```python
from build123d import *

# Parameters (mm, degrees)
SKETCH2_W           = 100
SKETCH2_H           = 72
BOSS_EXTRUDE1_DEPTH = 6.35
FILLET1_R           = 8
SKETCH4_R           = 6.25
SKETCH4_R_2         = 4
SKETCH4_R_3         = 3.15
SKETCH4_R_4         = 1.25
CUT_EXTRUDE9_DEPTH  = 124.386881393
SKETCH5_R           = 1.65
CUT_EXTRUDE11_DEPTH = 124.386881393
CHAMFER1_SIZE       = 1.5


with BuildPart() as part:
    # Sketch2 → Boss-Extrude1 (new body)
    with BuildSketch(Plane.XY):
        with Locations((50, 36)):
            Rectangle(SKETCH2_W, SKETCH2_H)
    extrude(amount=BOSS_EXTRUDE1_DEPTH)

    # Fillet1
    fillet1_edges = [part.edges().sort_by_distance(p)[0] for p in [
        (100, 0, 3.175),
        (0, 0, 3.175),
    ]]
    fillet(fillet1_edges, radius=FILLET1_R)

    # Sketch4 → Cut-Extrude9 (cut, through all)
    with BuildSketch(Plane.XY):
        with Locations((17.5, 14)):
            Circle(SKETCH4_R)
        with Locations((82.5, 14)):
            Circle(SKETCH4_R_2)
        with Locations((20, 57)):
            Circle(SKETCH4_R_3)
        with Locations((80, 57)):
            Circle(SKETCH4_R_3)
        with Locations((10, 45)):
            Circle(SKETCH4_R_4)
        with Locations((25, 45)):
            Circle(SKETCH4_R_4)
    extrude(amount=CUT_EXTRUDE9_DEPTH, mode=Mode.SUBTRACT)

    # Sketch5 → Cut-Extrude11 (cut, through all)
    with BuildSketch(Plane.XY.offset(6.35)):
        with Locations((10.126311132, 29.325110598)):
            Circle(SKETCH5_R)
        with Locations((36.565235622, 24.663214869)):
            Circle(SKETCH5_R)
        with Locations((19.308453246, 4.097382476)):
            Circle(SKETCH5_R)
    extrude(amount=-CUT_EXTRUDE11_DEPTH, mode=Mode.SUBTRACT)

    # Chamfer1
    chamfer1_edges = [part.edges().sort_by_distance(p)[0] for p in [
        (8.476311132, 29.325110598, 0),
        (8.476311132, 29.325110598, 6.35),
        (34.915235622, 24.663214869, 0),
        (34.915235622, 24.663214869, 6.35),
        (17.658453246, 4.097382476, 0),
        (17.658453246, 4.097382476, 6.35),
    ]]
    chamfer(chamfer1_edges, length=CHAMFER1_SIZE)


solid = part.part
```
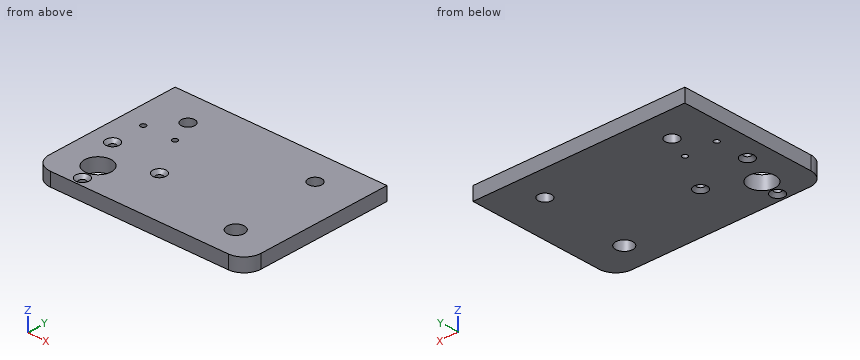
Geometry check sheet. Reference: the model listing, model coordinates, mm. Coordinates: 2 decimals unless noted, no trailing zeros. Order: outer loops, then holes, each group sorted by start corner. A loop starts at its lowest first (then second) coordinate and runs counter-clockwise, first axis right, second up. Notation, with made-up numbers: M 56.25,62 L 113.25,62 A20 ccw 113.25,98 Z; hole C 50.5,53 d3. An arc over 180 degrees is marked long. One line per question, with ' | ' between items. Start each with the question number.
Item 1: Material ranges on L1, parallel to X at y = 14, z = 4; L2, parallel to X at y = 57, z = 4.5; L3, parallel to Y at x = 10, z = 3.25, recorded low to high. Write a range as [from, to].
Item 2: Cross-section at C-C on z = 2.75. State how many separate pieces and enclosed holes the cut face has, then the cut area to 3 significant figures.
Item 3: Cross-section at D-D on x = 80. Enter the section's corners in (y, z), then the cut area to 3 significant figures.
Item 4: Cross-section at A-A on x = 25. Enter the section's corners in (y, z), then the cut area to 3 significant figures.
Item 5: Cross-section at B-B on y = 45. Enter the section's corners in (x, z), then the cut area to 3 significant figures.
Findings:
1) L1: x = [0, 11.25], [23.75, 78.5], [86.5, 100] | L2: x = [0, 16.85], [23.15, 76.85], [83.15, 100] | L3: y = [0, 27.68], [30.97, 43.75], [46.25, 72]
2) separate pieces: 1 | enclosed holes: 9 | area: 6,900 mm²
3) outline: M 0,0 L 10.88,0 L 10.88,6.35 L 0,6.35 Z; M 17.12,0 L 53.85,0 L 53.85,6.35 L 17.12,6.35 Z; M 60.15,0 L 72,0 L 72,6.35 L 60.15,6.35 Z | area: 378 mm²
4) outline: M 0,0 L 43.75,0 L 43.75,6.35 L 0,6.35 Z; M 46.25,0 L 72,0 L 72,6.35 L 46.25,6.35 Z | area: 441 mm²
5) outline: M 0,0 L 8.75,0 L 8.75,6.35 L 0,6.35 Z; M 11.25,0 L 23.75,0 L 23.75,6.35 L 11.25,6.35 Z; M 26.25,0 L 100,0 L 100,6.35 L 26.25,6.35 Z | area: 603 mm²
